Could you check a few things on this model? Use its own coordinates, in mm. A direction names the side the tool comes from. Give positions to 0.01 mm unless a question says otherwise; leave off trailing zeros. Loops run counter-clockwise (first coordinate to the right, second up) from the corner with the lowest first, then second, coordinate; pieces in that order, holes last. Notation, with made-up numbers: M 5.5,29 L 50.5,29 A33 cw 50.5,59 Z; hole C -39.5,-16.75 d8. An arc over 180 degrees is marked long. Use a Markdown table: item, result. Add a question column.
1) Suppose I cut it at D-D on x = 11.5. List the corners of the cut face in (y, z) for me.
2) Which directions (+Z, -Z, +X, -X, +Y, -Y) give clear straight access to the entire face, cutting with the end or side of a thin tool? Please do faces 1 (the cylindrical face through (40.293, -60.591, 17.776)), 2 (the cylindrical face through (26.793, -47.091, 34.74)), 3 (the cylindrical face through (-41.793, -62.091, 17.502)).
3) We'd pull the mould along Z, two halves only. Please class faces 4 (the flat face through (-33, -15, 34)), 5 (the flat face through (-31, -14, 35.5)), 6 (the cylindrical face through (41.591, -62.293, 17.502)): +Z half, -Z half, draft (parallel to the pull), parting line (faces both ways), or undercut.
4) Suppose I cut it at C-C on z = 26.5. List the corners of the cut face in (x, y) for me, and give its area (3 significant figures).
5) If I drill on line 1 along X through (y, z) = (28, 8); line 2 along Z through (x, y) = (37, -56.5); line 3 along Y through (x, z) = (-28.5, 13.5), over which ranges is the centre line in solid material (lowest first)? Write a range as [from, to].
6) Suppose I cut it at B-B on x = 0.5. List the corners of the cut face in (y, z) for me.
7) Suppose I cut it at A-A on y = -11. List the corners of the cut face in (x, z) for me.
8) Will these pins go through, and if not, where does the flat tip stop? pin 1 Ø1 at (x, z) = (-24.5, 6.5) entering from +Y; pin 2 Ø1.6 at (x, z) = (8, 35) entering from +Y; pin 3 Ø1 at (y, z) = (-30.5, 22) entering from +X; pin 4 Ø5 at (x, y) = (-36, 36) entering from -Z.
```python
from build123d import *

# Parameters (mm, degrees)
F0_W     = 64
F0_H     = 44.1964381933
F0_H_2   = 48.8035618067
F1_DEPTH = 2
F2_DEPTH = 34
F3_W     = 42
F3_H     = 13
F4_DEPTH = 5
F5_W     = 42
F5_H     = 15
F6_DEPTH = 5
F7_W     = 1.5
F7_H     = 73.5
F8_DEPTH = 1.5


with BuildPart() as f1:
    # F0 (on Top) → F1 (new body)
    with BuildSketch(Plane.XY):
        with BuildLine():
            Line((-31, -64.5), (31, -64.5))
            ThreePointArc((31, -64.5), (40.1923881554, -60.6923881554), (44, -51.5))
            Line((44, -51.5), (44, 64.5))
            Line((44, 64.5), (-44, 64.5))
            Line((-44, 64.5), (-44, -51.5))
            ThreePointArc((-44, -51.5), (-40.1923881554, -60.6923881554), (-31, -64.5))
        make_face()
        with Locations((0, -30.4017809033)):
            Rectangle(F0_W, F0_H, mode=Mode.SUBTRACT)
        with Locations((0, 28.0982190967)):
            Rectangle(F0_W, F0_H_2, mode=Mode.SUBTRACT)
    extrude(amount=F1_DEPTH)

    # F0 (on Top) → F2 (join)
    with BuildSketch(Plane.XY):
        with BuildLine():
            ThreePointArc((44, -51.5), (40.1923881554, -60.6923881554), (31, -64.5))
            Line((31, -64.5), (-31, -64.5))
            ThreePointArc((-31, -64.5), (-40.1923881554, -60.6923881554), (-44, -51.5))
            Line((-44, -51.5), (-44, 64.5))
            Line((-44, 64.5), (-45.5, 64.5))
            Line((-45.5, 64.5), (-45.5, -53))
            ThreePointArc((-45.5, -53), (-41.6923881554, -62.1923881554), (-32.5, -66))
            Line((-32.5, -66), (32.5, -66))
            ThreePointArc((32.5, -66), (41.6923881554, -62.1923881554), (45.5, -53))
            Line((45.5, -53), (45.5, 64.5))
            Line((45.5, 64.5), (44, 64.5))
            Line((44, 64.5), (44, -51.5))
        make_face()
    extrude(amount=F2_DEPTH)

    # F3 (on face) → F4 (cut)
    with BuildSketch(Plane.YZ.offset(45.5)):
        with Locations((-30, 27.5)):
            Rectangle(F3_W, F3_H)
    extrude(amount=-F4_DEPTH, mode=Mode.SUBTRACT)

    # F5 (on face) → F6 (cut)
    with BuildSketch(Plane.XZ.offset(66)):
        with Locations((-11.5, 26.5)):
            Rectangle(F5_W, F5_H)
    extrude(amount=-F6_DEPTH, mode=Mode.SUBTRACT)

    # F7 (on face) → F8 (join)
    with BuildSketch(Plane.XY.offset(34)):
        with BuildLine():
            Line((44, -9), (44, 64.5))
            Line((44, 64.5), (30.5, 64.5))
            Line((30.5, 64.5), (30.5, 51))
            Line((30.5, 51), (30.5, -38))
            ThreePointArc((30.5, -38), (26.6923881554, -47.1923881554), (17.5, -51))
            Line((17.5, -51), (-17.5, -51))
            ThreePointArc((-17.5, -51), (-26.6923881554, -47.1923881554), (-30.5, -38))
            Line((-30.5, -38), (-30.5, 51))
            Line((-30.5, 51), (-30.5, 64.5))
            Line((-30.5, 64.5), (-45.5, 64.5))
            Line((-45.5, 64.5), (-45.5, -53))
            ThreePointArc((-45.5, -53), (-41.6923881554, -62.1923881554), (-32.5, -66))
            Line((-32.5, -66), (32.5, -66))
            ThreePointArc((32.5, -66), (41.6923881554, -62.1923881554), (45.5, -53))
            Line((45.5, -53), (45.5, -9))
            Line((45.5, -9), (44, -9))
        make_face()
        with Locations((44.75, 27.75)):
            Rectangle(F7_W, F7_H)
    extrude(amount=F8_DEPTH)


solid = f1.part
```
Answer block:
| question | item | result |
|---|---|---|
| 1 | outline | M -66,0 L -52.5,0 L -52.5,2 L -64.5,2 L -64.5,34 L -51,34 L -51,35.5 L -66,35.5 Z; M -8.3,0 L 3.7,0 L 3.7,2 L -8.3,2 Z; M 52.5,0 L 64.5,0 L 64.5,2 L 52.5,2 Z |
| 2 | face 1 | +Y |
| 2 | face 2 | +Z, -Z, +Y |
| 2 | face 3 | +Z, -Z, -X, -Y |
| 3 | face 4 | undercut |
| 3 | face 5 | +Z half |
| 3 | face 6 | draft |
| 4 | outline | M -45.5,-53 A13 ccw -32.5,-66 L -32.5,-64.41 A13 cw -44,-51.5 L -44,64.5 L -45.5,64.5 Z; M 9.5,-66 L 32.5,-66 A13 ccw 45.5,-53 L 45.5,-51 L 44,-51 L 44,-51.5 A13 cw 31,-64.5 L 9.5,-64.5 Z; M 44,-9 L 45.5,-9 L 45.5,64.5 L 44,64.5 Z |
| 4 | area | 397 mm^2 |
| 5 | line 1 | x = [-45.5, -44], [44, 45.5] |
| 5 | line 2 | z = [0, 2], [34, 35.5] |
| 5 | line 3 | y = [-66, -64.5] |
| 6 | outline | M -66,0 L -52.5,0 L -52.5,2 L -64.5,2 L -64.5,19 L -66,19 Z; M -66,34 L -51,34 L -51,35.5 L -66,35.5 Z; M -8.3,0 L 3.7,0 L 3.7,2 L -8.3,2 Z; M 52.5,0 L 64.5,0 L 64.5,2 L 52.5,2 Z |
| 7 | outline | M -45.5,0 L -32,0 L -32,2 L -44,2 L -44,34 L -30.5,34 L -30.5,35.5 L -45.5,35.5 Z; M 30.5,34 L 45.5,34 L 45.5,35.5 L 30.5,35.5 Z; M 32,0 L 45.5,0 L 45.5,21 L 44,21 L 44,2 L 32,2 Z |
| 8 | pin 1 | stops at y = -64.5 |
| 8 | pin 2 | stops at y = -51 |
| 8 | pin 3 | stops at x = -44 |
| 8 | pin 4 | stops at z = 0 |
